Could you check a few things on this model? Use its own coordinates, in mm. A direction names the side the tool comes from. Give positions to 0.01 mm unless a question says otherwise; leave off trailing zeros. Write each loop counter-clockwise with the first axis right and the second up, starting at its lowest first coordinate (ties: lowest second). Pieces come first, ordered by that corner, then holes. Notation, with made-up numbers: (-1.5, -18) - (38.5, -18) arc R10 ccw to (38.5, -6) - close; hole circle Ø4 at (86, 31). An arc over 180 degrees is marked (long way). Use one line per item in the form item = value.
```python
from build123d import *

# Parameters (mm, degrees)
SKETCH1_W            = 60
SKETCH1_H            = 40
BOSS_EXTRUDE1_DEPTH  = 10
SKETCH2_W            = 6
SKETCH2_H            = 6
CUT_EXTRUDE1_DEPTH   = 73.801098893
LPATTERN1_COUNT      = 3
LPATTERN1_PITCH      = 15
LPATTERN1_COUNT_DIR2 = 2
LPATTERN1_PITCH_DIR2 = 15


with BuildPart() as part:
    # Sketch1 → Boss-Extrude1 (new body)
    with BuildSketch(Plane.XY):
        with Locations((30, 20)):
            Rectangle(SKETCH1_W, SKETCH1_H)
    extrude(amount=BOSS_EXTRUDE1_DEPTH)

    # Sketch2 → Cut-Extrude1 (cut, through all)
    with BuildSketch(Plane.XY):
        with Locations((9, 9)):
            Rectangle(SKETCH2_W, SKETCH2_H)
    cut_extrude1 = extrude(amount=CUT_EXTRUDE1_DEPTH, mode=Mode.SUBTRACT)

    # LPattern1: Cut-Extrude1 3 × 2
    with Locations(*[(i * LPATTERN1_PITCH, j * LPATTERN1_PITCH_DIR2, 0) for i in range(LPATTERN1_COUNT) for j in range(LPATTERN1_COUNT_DIR2) if (i, j) != (0, 0)]):
        add(cut_extrude1, mode=Mode.SUBTRACT)


solid = part.part
```
1. Which directions (+Z, -Z, +X, -X, +Y, -Y) give clear straight access to the entire face, cutting with the end or side of a thin tool? Please do faces 1 (the face through (9, 6, 5)), 2 (the face through (30, 20, 0)).
Response values:
face_1 = +Z, -Z
face_2 = -Z, +X, -X, +Y, -Y
2. If we mould it in two halves opening along X, with no side actions, what happens to faces 3 (the face through (39, 12, 5)), 4 (the face through (0, 20, 5)), 5 (the face through (30, 20, 10)), 6 (the face through (36, 24, 5))? For each: pulls with the +X half, pulls with the -X half, needs draft (parallel to the pull), parting line crosses it, or undercut.
Response values:
face_3 = undercut
face_4 = pulls with the -X half
face_5 = needs draft
face_6 = undercut
3. Imagine slicing it at B-B, the plane y = 7.5. List the corners of the cut face in (x, z) for me, and give its area (3 significant figures).
Response values:
outline = (0, 0) - (6, 0) - (6, 10) - (0, 10) - close; (12, 0) - (21, 0) - (21, 10) - (12, 10) - close; (27, 0) - (36, 0) - (36, 10) - (27, 10) - close; (42, 0) - (60, 0) - (60, 10) - (42, 10) - close
area = 420 mm²
4. Imagine slicing it at A-A, the plane x = 39.5. List the corners of the cut face in (y, z) for me, and give its area (3 significant figures).
Response values:
outline = (0, 0) - (6, 0) - (6, 10) - (0, 10) - close; (12, 0) - (21, 0) - (21, 10) - (12, 10) - close; (27, 0) - (40, 0) - (40, 10) - (27, 10) - close
area = 280 mm²
5. Imagine slicing it at C-C, the plane z = 8. List the corners of the cut face in (x, y) for me.
Response values:
outline = (0, 0) - (60, 0) - (60, 40) - (0, 40) - close; hole (6, 6) - (12, 6) - (12, 12) - (6, 12) - close; hole (6, 21) - (12, 21) - (12, 27) - (6, 27) - close; hole (21, 6) - (27, 6) - (27, 12) - (21, 12) - close; hole (21, 21) - (27, 21) - (27, 27) - (21, 27) - close; hole (36, 6) - (42, 6) - (42, 12) - (36, 12) - close; hole (36, 21) - (42, 21) - (42, 27) - (36, 27) - close
6. If I drill on line 1 (Y direction, x = 23.5, z = 1); line 2 (X direction, y = 23.5, z = 6.5), over which ranges is the centre line in solid material (lowest first)? Write a range as from..to.
Response values:
line_1 = 0..6, 12..21, 27..40
line_2 = 0..6, 12..21, 27..36, 42..60
